```python
from build123d import *

# Parameters (mm, degrees)
BOSS_EXTRUDE1_DEPTH     = 2
BOSS_EXTRUDE2_DEPTH     = 2
SKETCH10_R              = 1.5
CORTAR_EXTRUIR1_DEPTH   = 10
CROQUIS1_R              = 1.5
CORTAR_EXTRUIR2_DEPTH   = 10
SALIENTE_EXTRUIR1_DEPTH = 16


with BuildPart() as part:
    # Sketch1 → Boss-Extrude1 (new body)
    with BuildSketch(Plane.XY):
        with BuildLine():
            Line((0, 0), (0, -4))
            ThreePointArc((0, -4), (0.585786438, -5.414213562), (2, -6))
            Line((2, -6), (14, -6))
            ThreePointArc((14, -6), (15.414213562, -5.414213562), (16, -4))
            Line((16, -4), (16, 0))
            Line((16, 0), (0, 0))
        make_face()
    extrude(amount=BOSS_EXTRUDE1_DEPTH)

    # Sketch10 → Cortar-Extruir1 (cut)
    with BuildSketch(Plane(origin=(0, 0, 0), x_dir=(-1, 0, 0), z_dir=(0, 0, -1))):
        with Locations((-12, -3)):
            Circle(SKETCH10_R)
        with Locations((-4, -3)):
            Circle(SKETCH10_R)
    extrude(amount=-CORTAR_EXTRUIR1_DEPTH, mode=Mode.SUBTRACT)



with BuildPart() as body_2:
    # Sketch5 → Boss-Extrude2 (new body)
    with BuildSketch(Plane(origin=(0, 0, 0), x_dir=(1, 0, 0), z_dir=(0, 1, 0))):
        with BuildLine():
            Line((0, 0), (16, 0))
            ThreePointArc((16, 0), (8, 7.097527245), (0, 0))
        make_face()
    extrude(amount=BOSS_EXTRUDE2_DEPTH)

    # Croquis1 → Cortar-Extruir2 (cut)
    with BuildSketch(Plane(origin=(0, 2, 0), x_dir=(1, 0, 0), z_dir=(0, 1, 0))):
        with Locations(Location((8, 3.8, 0), (0, 0, 180))):
            Circle(CROQUIS1_R)
    extrude(amount=-CORTAR_EXTRUIR2_DEPTH, mode=Mode.SUBTRACT)


with BuildPart() as part_1:
    add(part.part)

    add(body_2.part)  # Saliente-Extruir1 merges body 2
    # Croquis2 → Saliente-Extruir1 (add)
    with BuildSketch(Plane.ZY):
        with BuildLine():
            Line((2, 0), (0, 0))
            Line((0, 0), (0, 2))
            ThreePointArc((0, 2), (1.414213562, 1.414213562), (2, 0))
        make_face()
    extrude(amount=-SALIENTE_EXTRUIR1_DEPTH)


solid = part_1.part
```
Input: part model. Units: mm. Frame: model coordinates. A direction names the side the tool comes from. Round coordinates to 2 decimals unless told otherwise and drop trailing zeros. Loops run counter-clockwise (first coordinate to the right, second up) from the corner with the lowest first, then second, coordinate; pieces in that order, holes last.
1) Section query B-B on y = -2.25. Return the cut outline in (x, z), plus the area to 3 significant figures.
Ans:
outline: (0, 0) - (2.7, 0) - (2.7, 2) - (0, 2) - close; (5.3, 0) - (10.7, 0) - (10.7, 2) - (5.3, 2) - close; (13.3, 0) - (16, 0) - (16, 2) - (13.3, 2) - close
area: 21.6 mm2
2) Pin query (flat end, axial travel): pin 1 (2.5 mm diameter, centred on x = 4, y = -3, fed in from -Z); pin 2 (2 mm diameter, centred on x = 5, y = -5, fed in from -Z); pin 3 (5 mm diameter, centred on x = 3.5, z = -3.5, fed in from -Y). Return the tip coordinate at first contact, or that it passes through.
Ans:
pin 1: passes through
pin 2: stops at z = 0
pin 3: stops at y = 0
3) Section query C-C on z = -3.8. Return the cut outline in (x, y), plus the area to 3 significant figures.
Ans:
outline: (1.5, 0) - (6.5, 0) - (6.5, 2) - (1.5, 2) - close; (9.5, 0) - (14.5, 0) - (14.5, 2) - (9.5, 2) - close
area: 20.0 mm2
4) Section query A-A on x = 4. Return the cut outline in (y, z), plus the area to 3 significant figures.
Ans:
outline: (-6, 0) - (-4.5, 0) - (-4.5, 2) - (-6, 2) - close; (-1.5, 0) - (0, 0) - (0, -6.03) - (2, -6.03) - (2, 0) arc R2 ccw to (0, 2) - (-1.5, 2) - close
area: 21.2 mm2
5) Material intervals for line 1 (Z direction, x = 7.5, y = -2); line 2 (X direction, y = 1, z = -2.75); line 3 (Y direction, x = 11.75, z = 0.75), sorted ascending.
Ans:
line 1: z = 0 to 2
line 2: x = 0.85 to 6.93, 9.07 to 15.15
line 3: y = -6 to -4.48, -1.52 to 1.85
6) Set-up query: faces 1 (the flat face through (8, 0, -2)), 2 (the cylindrical face through (7.89, 1.43, 1.4)). Return all of +Z, -Z, +X, -X, +Y, -Y with unobstructed straight access to the full face (end or side cutting, diameter ignored); none if empty.
Ans:
face 1: -Z, +X, -X, -Y
face 2: +Z, +X, -X, +Y
7) Section query D-D on y = -0.25. Return the cut outline in (x, z), plus the area to 3 significant figures.
Ans:
outline: (0, 0) - (16, 0) - (16, 2) - (0, 2) - close
area: 32.0 mm2
8) Pull-direction query (X, two-part tool) for faces 3 (the flat face through (0, -1, 1)), 4 (the flat face through (8, -3, 2)), 5 (the cylindrical face through (13.11, -1.99, 0.99)); classes: released by +X, released by -X, zero draft, split by the parting line, or undercut.
Ans:
face 3: released by -X
face 4: zero draft
face 5: undercut
